Read the model definition and answer for the solid it produces. Units are mm, in the model's axes. Face numbers are marked on the shaded views. Coordinates: 2 decimals unless noted, no trailing zeros. Write item = value, one per line.
from build123d import *

# Parameters (mm, degrees)
F0_W     = 240
F0_H     = 240
F2_W     = 220
F2_H     = 220
F4_W     = 210
F4_H     = 210
F5_DEPTH = 5
F7_DEPTH = 3


with BuildPart() as f3:
    # F0 (on Top) → F3 section 0
    with BuildSketch(Plane.XY):
        Rectangle(F0_W, F0_H)
    # F2 (on offset) → F3 section 1
    with BuildSketch(Plane.XY.offset(20)):
        Rectangle(F2_W, F2_H)
    loft()

    # F4 (on face) → F5 (cut)
    with BuildSketch(Plane.XY.offset(20)):
        Rectangle(F4_W, F4_H)
    extrude(amount=-F5_DEPTH, mode=Mode.SUBTRACT)

    # F6 (on face) → F7 (cut)
    with BuildSketch(Plane.XY.offset(15)):
        with BuildLine():
            ThreePointArc((-70, 75), (-78.5355339059, 78.5355339059), (-75, 70))
            Line((-75, 70), (-75, 75))
            Line((-75, 75), (-70, 75))
        make_face()
        with BuildLine():
            Line((-75, 75), (-75, 70))
            ThreePointArc((-75, 70), (-71.4644660941, 71.4644660941), (-70, 75))
            Line((-70, 75), (-75, 75))
        make_face()
        with BuildLine():
            ThreePointArc((70, 75), (71.4644660941, 71.4644660941), (75, 70))
            Line((75, 70), (75, 75))
            Line((75, 75), (70, 75))
        make_face()
        with BuildLine():
            Line((75, 75), (75, 70))
            ThreePointArc((75, 70), (78.5355339059, 71.4644660941), (80, 75))
            ThreePointArc((80, 75), (75, 80), (70, 75))
            Line((70, 75), (75, 75))
        make_face()
        with BuildLine():
            ThreePointArc((75, -70), (71.4644660941, -71.4644660941), (70, -75))
            Line((70, -75), (75, -75))
            Line((75, -75), (75, -70))
        make_face()
        with BuildLine():
            Line((75, -75), (70, -75))
            ThreePointArc((70, -75), (75, -80), (80, -75))
            ThreePointArc((80, -75), (78.5355339059, -71.4644660941), (75, -70))
            Line((75, -70), (75, -75))
        make_face()
        with BuildLine():
            Line((-75, -75), (-70, -75))
            ThreePointArc((-70, -75), (-71.4644660941, -71.4644660941), (-75, -70))
            Line((-75, -70), (-75, -75))
        make_face()
        with BuildLine():
            ThreePointArc((-75, -70), (-78.5355339059, -78.5355339059), (-70, -75))
            Line((-70, -75), (-75, -75))
            Line((-75, -75), (-75, -70))
        make_face()
    extrude(amount=-F7_DEPTH, mode=Mode.SUBTRACT)


solid = f3.part
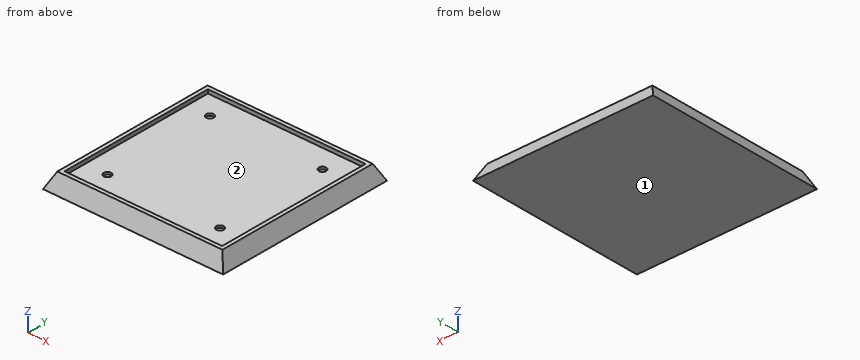
1) Determine the mould class of the marked faces 1 and 2 for opening direction X: pulls with the +X half, pulls with the -X half, needs draft (parallel to the pull), parting line crosses it, or undercut.
Returned:
face_1 = needs draft
face_2 = undercut
2) Straight lines are drawn through the part: line 1 along X through (y, z) = (75, 12.9); line 2 along Y through (x, z) = (-75, 13.95) (3 decimals); line 3 along Y through (x, z) = (-75, 13.4). For each, find the intervals that lie inside material, in ascending order. Write a range as from..to.
Returned:
line_1 = -113.55..-80, -70..70, 80..113.55
line_2 = -113.025..-80, -70..70, 80..113.025
line_3 = -113.3..-80, -70..70, 80..113.3
3) Flat-ended cylindrical pins translate along their axes: pin 1 Ø5 at (x, y) = (-75.5, 76) entering from +Z; pin 2 Ø1.5 at (y, z) = (-39.5, 18.5) entering from -X (3 decimals); pin 3 Ø5.5 at (x, z) = (-34.5, 17.5) entering from -Y (3 decimals). Find the tip coordinate at first contact, or state that the pin passes through.
Returned:
pin_1 = 12
pin_2 = -111.125
pin_3 = -112.625
